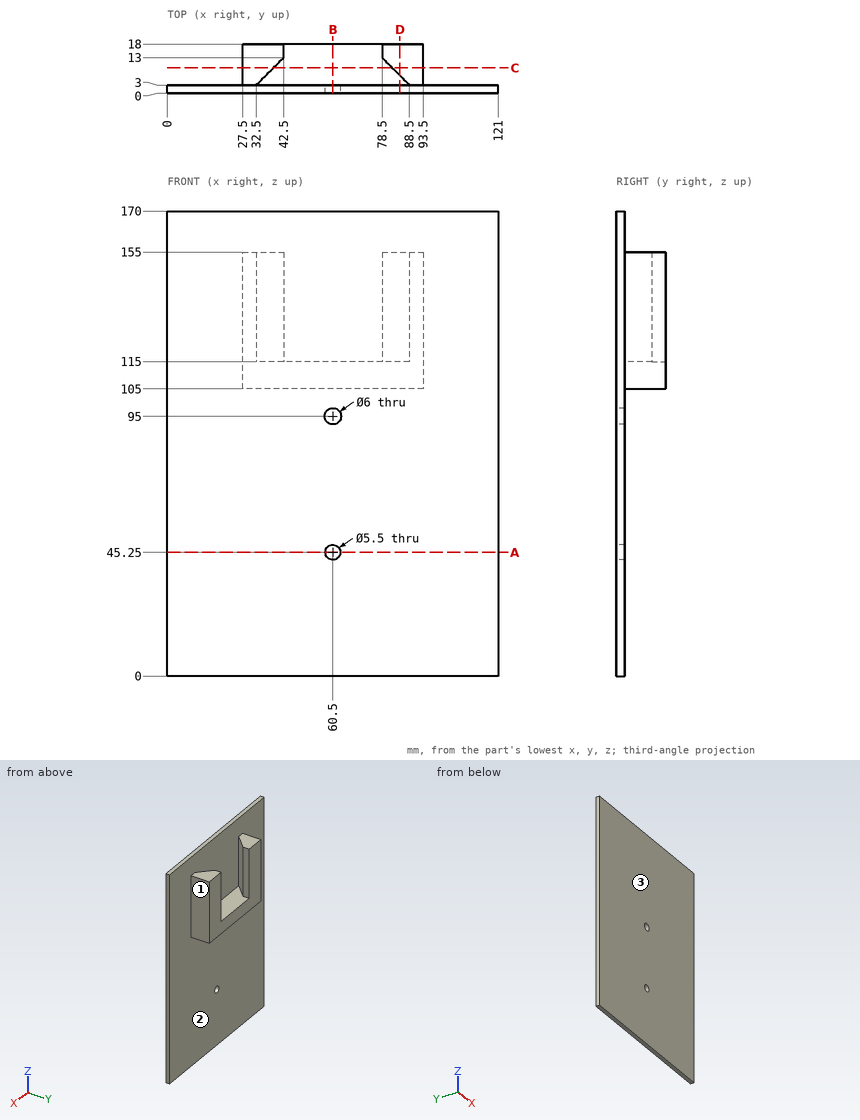
Drawing for the job (mm, zero at the part's lowest x, y, z). Round coordinates to 2 decimals unless told otherwise and drop trailing zeros. Loops run counter-clockwise (first coordinate to the right, second up) from the corner with the lowest first, then second, coordinate; pieces in that order, holes last. Notation, with made-up numbers: (30, -24) -> (75, -24) arc R30 ccw to (75, 4) -> close; hole circle Ø1 at (27, 73.25). An arc over 180 degrees is marked (long way). Answer in a Markdown table with one row per item.
Item 1: Mould opens along X. For the marked faces 1, 2 and 3 say: +X half, -X half, draft (parallel to the pull), parting line (faces both ways), or undercut.
Answers below:
| item | result |
|---|---|
| face 1 | +X half |
| face 2 | undercut |
| face 3 | draft |
Item 2: Saw through at C-C (y = 9.25). Write the cut outline in (x, z).
Answers below:
| item | result |
|---|---|
| outline | (27.5, 105) -> (93.5, 105) -> (93.5, 155) -> (82.25, 155) -> (82.25, 115) -> (38.75, 115) -> (38.75, 155) -> (27.5, 155) -> close |
Item 3: Pin check, flat tips, straight feed: pin 1 (1 mm diameter, centred on y = 5.5, z = 103.5, fed in from -X); pin 2 (4.5 mm diameter, centred on x = 35.5, y = 12.5, fed in from +Z); pin 3 (5 mm diameter, centred on y = 8.5, z = 147.5, fed in from -X); pin 4 (2.5 mm diameter, centred on y = 14.5, z = 139, fed in from +X). Stop position of each tip, or through.
Answers below:
| item | result |
|---|---|
| pin 1 | passes through |
| pin 2 | stops at z = 155 |
| pin 3 | stops at x = 27.5 |
| pin 4 | stops at x = 93.5 |
Item 4: Saw through at B-B (x = 60.5). Write the cut outline in (y, z).
Answers below:
| item | result |
|---|---|
| outline | (0, 0) -> (3, 0) -> (3, 42.5) -> (0, 42.5) -> close; (0, 48) -> (3, 48) -> (3, 92) -> (0, 92) -> close; (0, 98) -> (3, 98) -> (3, 105) -> (18, 105) -> (18, 115) -> (3, 115) -> (3, 170) -> (0, 170) -> close |
Item 5: Saw through at A-A (z = 45.25). Write the cut outline in (x, y).
Answers below:
| item | result |
|---|---|
| outline | (0, 0) -> (57.75, 0) -> (57.75, 3) -> (0, 3) -> close; (63.25, 0) -> (121, 0) -> (121, 3) -> (63.25, 3) -> close |
Item 6: Drill centre lines: L1, parallel to Z at x = 60.5, y = 1.7; L2, parallel to Y at x = 72, z = 87; L3, parallel to X at y = 6.5, z = 153.5. Where is each one in solid material? Low to high. Write a range as [from, to].
Answers below:
| item | result |
|---|---|
| L1 | z = [0, 42.5], [48, 92], [98, 170] |
| L2 | y = [0, 3] |
| L3 | x = [27.5, 36], [85, 93.5] |
Item 7: Saw through at D-D (x = 85). Write the cut outline in (y, z).
Answers below:
| item | result |
|---|---|
| outline | (0, 0) -> (3, 0) -> (3, 105) -> (18, 105) -> (18, 155) -> (6.5, 155) -> (6.5, 115) -> (3, 115) -> (3, 170) -> (0, 170) -> close |
